Build history of the part. All positions in model axes, mm. Face numbers are marked on the shaded views. A direction names the side the tool comes from. Round coordinates to 2 decimals unless told otherwise and drop trailing zeros. Order: outer loops, then holes, each group sorted by start corner. A loop starts at its lowest first (then second) coordinate and runs counter-clockwise, first axis right, second up. Notation, with made-up numbers: (49.25, -35.75) -> (83.25, -35.75) arc R37 cw to (83.25, 3.25) -> close; hole circle Ø1 at (60.5, 45). An arc over 180 degrees is marked (long way). Write item = value, one per line.
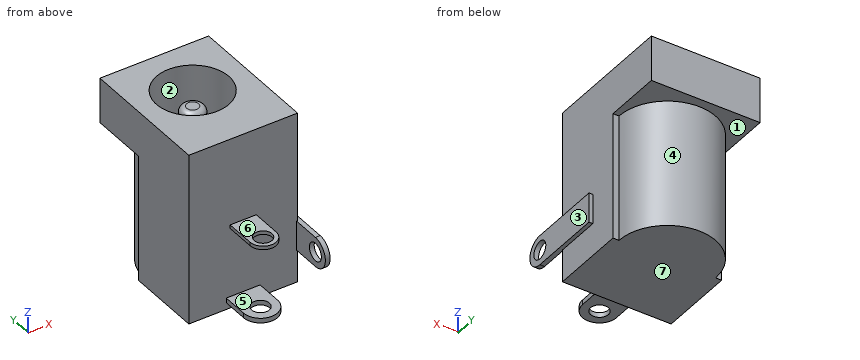
from build123d import *

# Parameters (mm, degrees)
SKETCH1_W           = 9.144
SKETCH1_H           = 11.176
BASE_EXTRUDE_DEPTH  = 3.81
BOSS_EXTRUDE1_DEPTH = 10.668
SKETCH3_R           = 3.048
CUT_EXTRUDE1_DEPTH  = 9.144
SKETCH4_R           = 1
EXTRUDE1_DEPTH      = 7.804
FILLET1_R           = 0.5
SKETCH5_R           = 0.75
EXTRUDE2_DEPTH      = 0.2
SKETCH6_R           = 0.75
EXTRUDE3_DEPTH      = 0.15
SKETCH7_R           = 0.75
EXTRUDE4_DEPTH      = 0.2


with BuildPart() as part:
    # Sketch1 → Base-Extrude (new body)
    with BuildSketch(Plane.XY):
        with Locations((0, 5.588)):
            Rectangle(SKETCH1_W, SKETCH1_H)
    extrude(amount=-BASE_EXTRUDE_DEPTH)

    # Sketch2 → Boss-Extrude1 (add)
    with BuildSketch(Plane(origin=(0, 0, -3.81), x_dir=(-1, 0, 0), z_dir=(0, 0, -1))):
        with BuildLine():
            Line((-4.572, 0), (-4.572, 6.35))
            Line((-4.572, 6.35), (-4.064, 6.35))
            ThreePointArc((-4.064, 6.35), (0, 10.414), (4.064, 6.35))
            Line((4.064, 6.35), (4.572, 6.35))
            Line((4.572, 6.35), (4.572, 0))
            Line((4.572, 0), (-4.572, 0))
        make_face()
    extrude(amount=BOSS_EXTRUDE1_DEPTH)

    # Sketch3 → Cut-Extrude1 (cut)
    with BuildSketch(Plane.XY):
        with Locations((0, 6.35)):
            Circle(SKETCH3_R)
    extrude(amount=-CUT_EXTRUDE1_DEPTH, mode=Mode.SUBTRACT)

    # Sketch4 → Extrude1 (add)
    with BuildSketch(Plane.XY.offset(-9.144)):
        with Locations((0, 6.35)):
            Circle(SKETCH4_R)
    extrude(amount=EXTRUDE1_DEPTH)

    # Fillet1
    fillet1_edges = [part.edges().sort_by_distance(p)[0] for p in [
        (-1, 6.35, -1.34),
    ]]
    fillet(fillet1_edges, radius=FILLET1_R)

    # Sketch5 → Extrude2 (add, symmetric)
    with BuildSketch(Plane(origin=(4.7, 0, 0), x_dir=(0, 0, -1), z_dir=(1, 0, 0))):
        with BuildLine():
            Line((11.75, 3.83), (11.75, -2.35))
            ThreePointArc((11.75, -2.35), (10.5, -3.6), (9.25, -2.35))
            Line((9.25, -2.35), (9.25, 3.83))
            Line((9.25, 3.83), (11.75, 3.83))
        make_face()
        with Locations((10.5, -2.35)):
            Circle(SKETCH5_R, mode=Mode.SUBTRACT)
    extrude(amount=EXTRUDE2_DEPTH, both=True)

    # Sketch6 → Extrude3 (add, symmetric)
    with BuildSketch(Plane(origin=(0, 0, -7.5), x_dir=(-1, 0, 0), z_dir=(0, 0, 1))):
        with BuildLine():
            Line((-1.1, 0), (-1.1, 2.5))
            ThreePointArc((-1.1, 2.5), (0, 3.6), (1.1, 2.5))
            Line((1.1, 2.5), (1.1, 0))
            Line((1.1, 0), (-1.1, 0))
        make_face()
        with Locations((0, 2.5)):
            Circle(SKETCH6_R, mode=Mode.SUBTRACT)
    extrude(amount=EXTRUDE3_DEPTH, both=True)

    # Sketch7 → Extrude4 (add, symmetric)
    with BuildSketch(Plane.XY.offset(-13.7)):
        with BuildLine():
            Line((1.425, 0), (1.425, -2.175))
            ThreePointArc((1.425, -2.175), (0, -3.6), (-1.425, -2.175))
            Line((-1.425, -2.175), (-1.425, 0))
            Line((-1.425, 0), (1.425, 0))
        make_face()
        with Locations((0, -2.175)):
            Circle(SKETCH7_R, mode=Mode.SUBTRACT)
    extrude(amount=EXTRUDE4_DEPTH, both=True)


solid = part.part
Q1. Cut at C-C, the plane y = 2.75. List the corners of the cut face in (x, z).
Check values:
outline = (-4.57, -14.48) -> (4.57, -14.48) -> (4.57, -11.75) -> (4.9, -11.75) -> (4.9, -9.25) -> (4.57, -9.25) -> (4.57, 0) -> (-4.57, 0) -> close
Q2. Cut at B-B, the plane z = -10.5. List the corners of the cut face in (x, y), and give its area (3 significant figures).
Check values:
outline = (-4.57, 0) -> (4.5, 0) -> (4.5, -1.6) -> (4.9, -1.6) -> (4.9, 3.83) -> (4.57, 3.83) -> (4.57, 6.35) -> (4.06, 6.35) arc R4.06 ccw to (-4.06, 6.35) -> (-4.57, 6.35) -> close; (4.5, -3.6) -> (4.9, -3.6) -> (4.9, -3.1) -> (4.5, -3.1) -> close
area = 86.1 mm²
Q3. Cut at D-D, the plane y = -0.5. List the corners of the cut face in (x, z) (3 decimals).
Check values:
outline = (-1.425, -13.9) -> (1.425, -13.9) -> (1.425, -13.5) -> (-1.425, -13.5) -> close; (-1.1, -7.65) -> (1.1, -7.65) -> (1.1, -7.35) -> (-1.1, -7.35) -> close; (4.5, -11.75) -> (4.9, -11.75) -> (4.9, -9.25) -> (4.5, -9.25) -> close
Q4. Probe probe 1 along Y at (x, z) = (0, -4.25); probe 2 along Y at (x, z) = (0, -7.4); probe 3 along Y at (x, z) = (0, -13.65) (3 decimals). List the from-to ranges inside material, lowest first.
Check values:
probe_1 = 0 to 3.3, 5.35 to 7.35, 9.4 to 10.41
probe_2 = -3.6 to -3.25, -1.75 to 3.3, 5.35 to 7.35, 9.4 to 10.41
probe_3 = -3.6 to -2.925, -1.425 to 10.414
Q5. Flat gauge pins, fed straight in: pin 1 (1.8 mm diameter, centred on x = 0, y = -2.5, fed in from -Z); pin 2 (5 mm diameter, centred on y = 6.5, z = -12, fed in from +X); pin 3 (1.1 mm diameter, centred on x = 0, y = 6, fed in from +Z); pin 4 (1.4 mm diameter, centred on y = -2.35, z = -10.5, fed in from -X). Where does each tip first touch, or does it go through?
Check values:
pin_1 = -13.9
pin_2 = 4.57
pin_3 = -1.34
pin_4 = through
Q6. Mould opens along Z. For the marked faces 4, 5, 6 and 7 say: released by +Z, released by -Z, zero draft, split by the parting line, or undercut.
Check values:
face_4 = zero draft
face_5 = undercut
face_6 = released by +Z
face_7 = released by -Z
Q7. Which spindle directions (+Z, -Z, +X, -X, +Y, -Y) get a long thin tool onto all of the face, cutting with end or side? Do the marked faces 1, 2 and 3. Say none if no direction does.
Check values:
face_1 = -Z, +Y
face_2 = +Z
face_3 = +Z, -Z, +X, +Y, -Y
Q8. Cut at A-A, the plane z = -4. List the corners of the cut face in (x, y), and give its area (3 significant figures).
Check values:
outline = (-4.57, 0) -> (4.57, 0) -> (4.57, 6.35) -> (4.06, 6.35) arc R4.06 ccw to (-4.06, 6.35) -> (-4.57, 6.35) -> close; circle Ø2 at (0, 6.35); hole circle Ø6.1 at (0, 6.35)
area = 58.0 mm²
